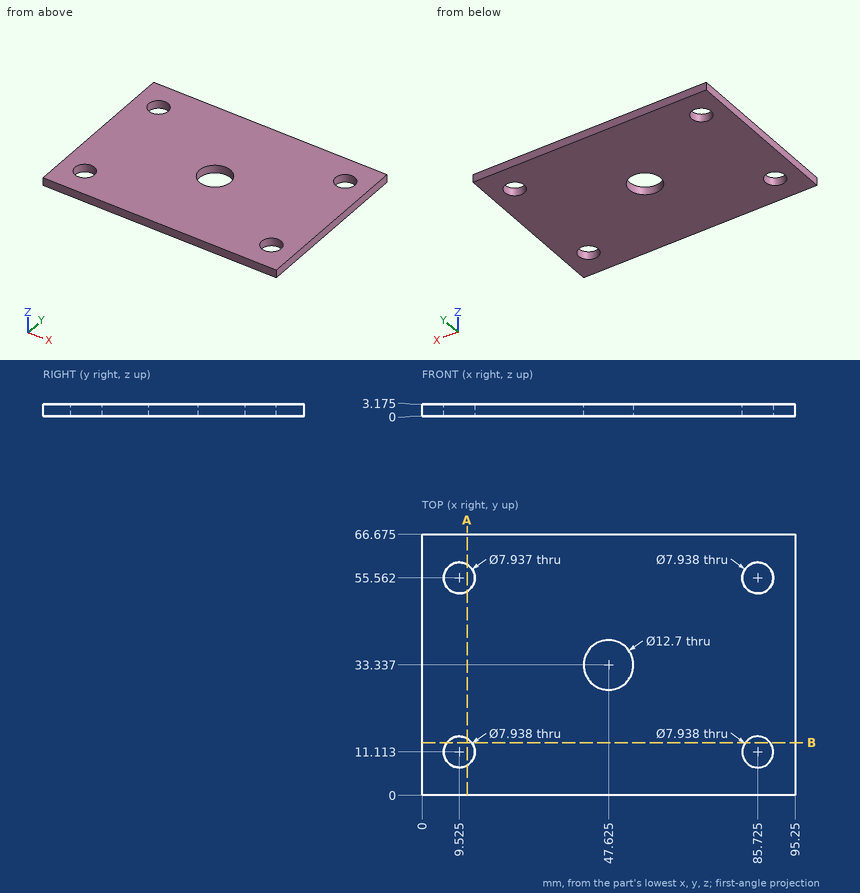
The figure shows three views and two pictorial views of one solid part (mm, origin at its lowest corner). Answer the questions. Round coordinates to 2 decimals unless told otherwise and drop trailing zeros. Write each loop counter-clockwise with the first axis right and the second up, starting at its lowest first coordinate (ties: lowest second). Pieces come first, ordered by that corner, then holes. Notation, with made-up numbers: (39.5, 61) - (52.5, 61) arc R4 ccw to (52.5, 67) - close; hole circle Ø2 at (36.25, 47). An arc over 180 degrees is marked (long way). One line per question, with ' | ' between items. Start each with the question number.
1. Find the intervals of material crossed by probe 1 along Y at (x, z) = (6, 1.1) (1 decimal); probe 2 along Y at (x, z) = (45, 0.45) (1 decimal); probe 3 along X at (y, z) = (32, 0.95), in increasing order. Write a range as [from, to].
2. Section B-B (y = 13.5) is taken. Give the number of separate pieces and of enclosed holes in the cut face, and give its area (3 significant figures).
3. Section A-A (x = 11.5) is taken. Determine the outline of the cut face in (y, z) (1 decimal), and give its area (3 significant figures).
Filled in:
1) probe 1: [0, 9.3], [12.9, 53.7], [57.4, 66.7] | probe 2: [0, 27.6], [39.1, 66.7] | probe 3: [0, 41.42], [53.83, 95.25]
2) separate pieces: 3 | enclosed holes: 0 | area: 262 mm²
3) outline: (0, 0) - (7.7, 0) - (7.7, 3.2) - (0, 3.2) - close; (14.6, 0) - (52.1, 0) - (52.1, 3.2) - (14.6, 3.2) - close; (59, 0) - (66.7, 0) - (66.7, 3.2) - (59, 3.2) - close | area: 168 mm²
